Autodesk Inventor part; units mm, degrees
ref_plane "Work Plane1" through (0, 0, -15) normal (0, 0, 1) x (1, 0, 0)
ref_plane "YZ Plane" through (0, 0, 0) normal (1, 0, 0) x (0, 1, 0)
ref_plane "XZ Plane" through (0, 0, 0) normal (0, 1, 0) x (-1, 0, 0)
sketch "Sketch1" plane through (0, 0, 0) normal (0, 0, 1) x (1, 0, 0)
  line L0 (0, 0) -> (25, 0)
  line L1 (25, 0) -> (25, 40)
  line L2 (25, 40) -> (0, 40)
  line L3 (0, 40) -> (0, 0)
  dimension "d1" = 25
  dimension "d2" = 40
  dimension "d3" = 25
extrude "Extrusion1" add sketch "Sketch1" against normal blind 30
sketch "Sketch2" plane through (25, 0, 0) normal (1, 0, 0) x (0, 0, -1)
  line L0 (0, 0) -> (30, 0)
  circle A0 centre (15, 6.56) radius 2.46
extrude "Extrusion2" cut sketch "Sketch2" against normal blind 30
sketch "Sketch3" plane through (0, 0, 0) normal (-1, 0, 0) x (0, 0, 1)
  line L0 (0, 0) -> (-30, 0)
  line L1 (-25.05, 0) -> (-4.95, 0)
  line L2 (-4.95, 0) -> (-4.95, 33.12)
  line L3 (-4.95, 33.12) -> (-25.05, 33.12)
  line L4 (-25.05, 33.12) -> (-25.05, 0)
  dimension "d11" = 20.1
extrude "Extrusion3" cut sketch "Sketch3" against normal blind 20
sketch "Sketch4" plane through (0, 0, 0) normal (0, -1, 0) x (1, 0, 0)
  line L0 (20, -4.95) -> (20, -25.05)
  line L1 (20, -15) -> (25, -15)
  line L2 (25, 0) -> (25, -30)
  line L3 (20, -8.025) -> (25, -8.025)
  line L4 (25, -8.025) -> (25, -21.975)
  line L5 (25, -21.975) -> (20, -21.975)
  line L6 (20, -21.975) -> (20, -8.025)
  line L7 (20, -8.025) -> (25, -21.975) construction
  line L8 (25, -8.025) -> (20, -21.975) construction
  line L9 (25, -12.54) -> (25, -17.46)
  point P0 (0, 0)
  point P1 (22.5, -15)
  dimension "d14" = 13.95
extrude "Extrusion4" add sketch "Sketch4" along normal blind 15
sketch "Sketch5" plane through (20, 0, 0) normal (-1, 0, 0) x (0, 0, 1)
  circle A0 centre (-15, 6.56) radius 2.46
  circle A1 centre (-15, 6.56) radius 4.7025
  circle A2 centre (-15, 6.56) radius 2.46
  circle A3 centre (-15, 6.56) radius 2.46
  point P0 (0, 0)
  dimension "d17" = 9.405
extrude "Extrusion5" cut sketch "Sketch5" against normal blind 2.1
sketch "Sketch6" plane through (25, 0, 0) normal (1, 0, 0) x (0, 0, -1)
  circle A0 centre (15, 6.56) radius 4.7025
  line L0 (15, 6.56) -> (15, 23.56)
  circle A1 centre (15, 23.56) radius 2.46
  point P0 (0, 0)
  dimension "d20" = 17
  dimension "d21" = 4.92
extrude "Extrusion6" cut sketch "Sketch6" against normal blind 10 contours A1
sketch "Sketch7" plane through (20, 0, 0) normal (-1, 0, 0) x (0, 0, 1)
  circle A0 centre (-15, 23.56) radius 2.46
  circle A1 centre (-15, 23.56) radius 4.7025
  point P0 (0, 0)
  dimension "d24" = 9.405
extrude "Extrusion7" cut sketch "Sketch7" against normal blind 2.1
sketch "Sketch9" plane through (25, 0, 0) normal (1, 0, 0) x (0, 0, -1)
  circle A0 centre (15, 6.56) radius 2.46
  circle A1 centre (15, 6.56) radius 2.46
  circle A2 centre (15, 23.56) radius 2.46
  circle A3 centre (15, 23.56) radius 2.46
  line L0 (30, 40) -> (30, 0)
  line L1 (30, 0) -> (30, 40)
  line L2 (30, 40) -> (0, 40)
  line L3 (0, 40) -> (0, 0)
  line L4 (0, 0) -> (8.025, 0)
  line L5 (21.975, 0) -> (21.975, -15)
  line L6 (21.975, -15) -> (8.025, -15)
  line L7 (8.025, -15) -> (8.025, 0)
  line L8 (0, 0) -> (8.025, 0)
  line L9 (21.975, 0) -> (30, 0)
extrude "Extrusion8" add sketch "Sketch9" along normal blind 5
sketch "Sketch10" plane through (0, 40, 0) normal (0, 1, 0) x (1, 0, 0)
  line L0 (0, 30) -> (30, 30)
  line L1 (30, 0) -> (0, 0)
  line L2 (0, 30) -> (30, 30)
  line L3 (30, 30) -> (30, 0)
  line L4 (30, 0) -> (0, 0)
  line L5 (0, 0) -> (0, 30)
extrude "Extrusion9" add sketch "Sketch10" along normal blind 30
sketch "Sketch12" plane through (30, 0, 0) normal (1, 0, 0) x (0, 0, -1)
  circle A0 centre (15, 6.56) radius 2.46
  line L0 (15, 6.56) -> (15, 15.06)
  circle A1 centre (15, 15.06) radius 2.525
  point P0 (0, 0)
  dimension "d31" = 8.5
  dimension "d33" = 5.05
extrude "Extrusion10" cut sketch "Sketch12" against normal blind 30 contours A1
sketch "Sketch14" plane through (0, 0, 0) normal (0, 0, 1) x (1, 0, 0)
  line L0 (30, 70) -> (0, 70)
  line L1 (0, 100) -> (-8, 100)
  line L2 (30, 0) -> (30, 70)
  line L3 (30, 118) -> (30, 70)
  line L4 (30, 105) -> (30, 100)
  line L5 (0, 70) -> (30, 70)
  line L6 (0, 70) -> (0, 100)
  line L7 (15, 136) -> (30, 118)
  line L8 (-8, 136) -> (15, 136)
  line L9 (-8, 100) -> (-8, 136)
  point P0 (0, 0)
  dimension "d47" = 30
extrude "Extrusion12" add sketch "Sketch14" against normal blind 30
sketch "Sketch15" plane through (0, 0, -25.05) normal (-1, 0, 0) x (0, 0, 1)
  line L0 (0, 33.12) -> (20.1, 33.12)
  line L1 (20.1, 33.12) -> (20.1, 0)
  line L2 (0, 33.12) -> (20.1, 33.12)
  line L3 (20.1, 33.12) -> (20.1, 31.1)
  line L4 (20.1, 31.1) -> (0, 31.1)
  line L5 (0, 31.1) -> (0, 33.12)
  point P0 (25.05, 0)
  dimension "d57" = 2.02
extrude "Extrusion13" add sketch "Sketch15" against normal blind 20
sketch "Sketch23" plane through (0, 0, 0) normal (0, 0, 1) x (1, 0, 0)
  line L0 (0, 100) -> (-8, 100)
  line L1 (-8, 136) -> (15, 136)
  line L2 (-8, 136) -> (15, 136)
  line L3 (30, 118) -> (15, 136)
  line L4 (15, 136) -> (30, 118)
  line L5 (30, 118) -> (30, 93)
  line L6 (30, 0) -> (30, 118)
  line L7 (30, 93) -> (0, 93)
  line L8 (0, 93) -> (0, 100)
  line L9 (-8, 100) -> (0, 100)
  line L10 (15, 136) -> (-8, 136)
  line L11 (-8, 136) -> (-8, 100)
  point P0 (0, 0)
  point P1 (-2, 102)
  point P2 (4, 118)
  point P3 (-2, 134)
  dimension "d85" = 25
extrude "Extrusion14" add sketch "Sketch23" along normal blind 15
ref_plane "Work Plane1" through (0, 0, -15) normal (0, 0, 1) x (1, 0, 0)
mirror "Mirror1" about plane through (0, 0, -15) normal (0, 0, 1) of "Extrusion14"
sketch "Sketch27" plane through (-8, 136, 15) normal (0, 1, 0) x (1, 0, 0)
  line L0 (0, 60) -> (0, 0)
  line L1 (0, 30) -> (0, 7.5)
  line L2 (8, 60) -> (8, 0)
  line L3 (0, 52.5) -> (0, 30)
  line L4 (0, 52.5) -> (5, 30)
  line L5 (5, 30) -> (0, 7.5)
  point P0 (8, 15)
  dimension "d94" = 22.5
extrude "Extrusion16" cut sketch "Sketch27" against normal through all
properties part number "orien_b_40mm"
Work out the finished part from the listing and answer in its coordinate system (mm). A direction names the side the tool comes from. Coordinates: 2 decimals unless noted, no trailing zeros. Loops run counter-clockwise (first coordinate to the right, second up) from the corner with the lowest first, then second, coordinate; pieces in that order, holes last. Notation, with made-up numbers: M -31.5,5.5 L 8.5,5.5 A23 cw 8.5,35.5 Z; hole C 87.5,74.25 d2. An arc over 180 degrees is marked long. Answer in a Markdown table with one row per item. Add a question column.
1. Find section B-B, the plane x = 27. Write down the section's boundary in (y, z) (3 decimals).
2. Find section A-A, the plane y = 15.06. Write down the section's boundary in (x, z) (3 decimals).
3. Consider L1, parallel to Z at x = 23, y = 15.06 (3 decimals); L2, parallel to Z at x = 9.5, y = 27.5; L3, parallel to Y at x = 26, z = -15 (3 decimals). Determine where each line is inside the solid, lowest interval first.
4. Find section C-C, the plane x = 12.5. Write down the section's boundary in (y, z), then the cut area to 3 significant figures.
5. The mould has two halves that part along Z. Classify faces 6 (the flat face through (30, 65, -15)), 7 (the flat face through (15, 47, 0)), 8 (the flat face through (10, 15, -4.95)): pulls with the +Z half, pulls with the -Z half, needs draft (parallel to the pull), parting line crosses it, or undercut.
6. A tool of negligible diameter and unlimited length cuts with its end or side. For faces 1 (the flat face through (20, 8, -20)), 2 (the flat face through (15, 93, -37)), 3 (the flat face through (25, -8, -8.025)), 4 (the flat face through (-5.465, 118.252, -3.908)), 5 (the cylindrical face through (21.035, 27.525, -12.472)), from which of +Z, -Z, +X, -X, +Y, -Y can it reach the whole face along a straight path? Write none if from no direction.
7. Flat-ended cylindrical pins translate along their axes: P1, Ø12, axis at y = 60.5, z = -27.5, coming from the -X side; P2, Ø5.5, axis at y = 6.56, z = -15, coming from the +X side; P3, Ø7.5, axis at y = 25, z = -16.5, coming from the -X side; P4, Ø5, axis at x = 9.5, y = 52, coming from the -Z side. Find the tip coordinate at first contact, or state that the pin passes through.
8. Find section D-D, the plane z = -35. Write down the section's boundary in (x, y).
Reported:
| question | item | result |
|---|---|---|
| 1 | outline | M -15,-21.975 L 0,-21.975 L 0,-30 L 93,-30 L 93,-45 L 121.6,-45 L 121.6,15 L 93,15 L 93,0 L 0,0 L 0,-8.025 L -15,-8.025 Z; hole C 6.56,-15 d4.92; hole C 15.06,-15 d5.05; hole C 23.56,-15 d4.92 |
| 2 | outline | M 0,-30 L 30,-30 L 30,-17.525 L 20,-17.525 L 20,-25.05 L 0,-25.05 Z; M 0,-4.95 L 20,-4.95 L 20,-12.475 L 30,-12.475 L 30,0 L 0,0 Z |
| 3 | L1 | z = -30 to -17.525, -12.475 to 0 |
| 3 | L2 | z = -30 to -25.05, -4.95 to 0 |
| 3 | L3 | y = -15 to 4.1, 9.02 to 12.535, 17.585 to 21.1, 26.02 to 122.8 |
| 4 | outline | M 0,-30 L 93,-30 L 93,-45 L 136,-45 L 136,15 L 93,15 L 93,0 L 0,0 L 0,-4.95 L 31.1,-4.95 L 31.1,-25.05 L 0,-25.05 Z |
| 4 | area | 4,740 mm^2 |
| 5 | face 6 | needs draft |
| 5 | face 7 | pulls with the +Z half |
| 5 | face 8 | undercut |
| 6 | face 1 | -X, -Y |
| 6 | face 2 | -Z, +X, -X, -Y |
| 6 | face 3 | +Z, +X, -X, -Y |
| 6 | face 4 | -X, +Y, -Y |
| 6 | face 5 | -X |
| 7 | P1 | stops at x = 0 |
| 7 | P2 | stops at x = 30 |
| 7 | P3 | stops at x = 20 |
| 7 | P4 | stops at z = -30 |
| 8 | outline | M -7.44,100 L 0,100 L 0,93 L 30,93 L 30,118 L 15,136 L -7.44,136 Z |
